```python
from build123d import *

# Parameters (mm, degrees)
F1_DEPTH    = 7.5
F2_W        = 16.1389429122
F2_H        = 16.083650291
F3_DEPTH    = 3
F4_D        = 3.5
F5_T1_DEPTH = 48.2954240112
F6_R        = 5


# Not quite as in the source:
# - a fillet or chamfer that OpenCascade refuses, or shapes differently, is made with other operations: its cross-section is extruded or revolved along the edge and cut away or added


with BuildPart() as f1:
    # F0 (on Top) → F1 (new body)
    with BuildSketch(Plane.XY):
        with BuildLine():
            ThreePointArc((-4.3675557451, -3.9293869513), (0, 5.875), (4.3675557451, -3.9293869513))
            Line((4.3675557451, -3.9293869513), (8.0694714561, -7.2599132545))
            Line((8.0694714561, -7.2599132545), (8.0694714561, 7.2599132545))
            Line((8.0694714561, 7.2599132545), (-8.0694714561, 7.2599132545))
            Line((-8.0694714561, 7.2599132545), (-8.0694714561, -7.2599132545))
            Line((-8.0694714561, -7.2599132545), (-4.3675557451, -3.9293869513))
        make_face()
    extrude(amount=F1_DEPTH)

    # F2 (on face) → F3 (join)
    with BuildSketch(Plane(origin=(0, 7.2599132545, 0), x_dir=(-1, 0, 0), z_dir=(0, 1, 0))):
        with Locations((0, -8.0418251455)):
            Rectangle(F2_W, F2_H)
        with BuildLine():
            Line((1.5, -5.9119383805), (1.5, -11.5))
            ThreePointArc((1.5, -11.5), (0, -13), (-1.5, -11.5))
            Line((-1.5, -11.5), (-1.5, -5.9119383805))
            ThreePointArc((-1.5, -5.9119383805), (0, -4.4119383805), (1.5, -5.9119383805))
        make_face(mode=Mode.SUBTRACT)
        with Locations((0, 8.0418251455)):
            Rectangle(F2_W, F2_H)
    extrude(amount=F3_DEPTH)

    # F4 (through all)
    with Locations(Plane(origin=(0, 7.2599132545, 0), x_dir=(-1, 0, 0), z_dir=(0, -1, 0))):
        with Locations((0, -11.5)):
            Hole(F4_D / 2)

    # F5: fillet of radius 5 on 2 edges, made by hand

    # F5_s2 → F5_t1 (cut)
    with BuildSketch(Plane.XY.offset(-20.3977120056)):
        with BuildLine():
            ThreePointArc((-8.0694714561, 0.8991715477), (-7.0374949846, -2.1429969679), (-4.3675557451, -3.9293869513))
            Line((-4.3675557451, -3.9293869513), (-8.0694714561, -7.2599132545))
            Line((-8.0694714561, -7.2599132545), (-8.0694714561, 0.8991715477))
        make_face()
        with BuildLine():
            ThreePointArc((8.0694714561, 0.8991715477), (7.0374949846, -2.1429969679), (4.3675557451, -3.9293869513))
            Line((4.3675557451, -3.9293869513), (8.0694714561, -7.2599132545))
            Line((8.0694714561, -7.2599132545), (8.0694714561, 0.8991715477))
        make_face()
    extrude(amount=F5_T1_DEPTH, mode=Mode.SUBTRACT)

    # F6
    f6_edges = [f1.edges().sort_by_distance(p)[0] for p in [
        (-8.069471, 8.759913, 16.08365),
        (8.069471, 8.759913, 16.08365),
        (8.069471, 8.759913, -16.08365),
        (-8.069471, 8.759913, -16.08365),
    ]]
    fillet(f6_edges, radius=F6_R)


solid = f1.part
```
Geometry: final body of the model. Coordinates: model frame, mm. A direction names the side the tool comes from. Round coordinates to 2 decimals unless told otherwise and drop trailing zeros. Loops run counter-clockwise (first coordinate to the right, second up) from the corner with the lowest first, then second, coordinate; pieces in that order, holes last. Notation, with made-up numbers: (33, 52) -> (48, 52) arc R26 cw to (48, 86) -> close; hole circle Ø10 at (69, 3.25). An arc over 180 degrees is marked (long way). Write each question's results on one line, items separated by ' | '.
Item 1: Set-up query: faces 1 (the face through (-0.19, 5.87, 3.7)), 2 (the face through (0.033, 8.739, -4.412)), 3 (the face through (-2, 7.26, -8)). Return all of +Z, -Z, +X, -X, +Y, -Y with unobstructed straight access to the full face (end or side cutting, diameter ignored); none if empty.
Answers below:
face 1: +Z, -Z | face 2: +Y, -Y | face 3: -Z, +X, -X, -Y
Item 2: Cut plane A-A on x = 0. Return the cut outline in (y, z) (3 decimals).
Answers below:
outline: (5.875, 0) -> (7.26, 0) -> (7.26, -4.412) -> (10.26, -4.412) -> (10.26, 9.75) -> (7.26, 9.75) -> (7.26, 7.5) -> (5.875, 7.5) -> close; (7.26, -16.084) -> (10.26, -16.084) -> (10.26, -13) -> (7.26, -13) -> close; (7.26, 13.25) -> (10.26, 13.25) -> (10.26, 16.084) -> (7.26, 16.084) -> close
Item 3: Line query: probe 1 along Z at (x, y) = (0, 9.5); probe 2 along Z at (x, y) = (4, 6.5); probe 3 along Y at (x, z) = (2, 13.5). Output: solid intervals per line, ascending. Write a range as [from, to].
Answers below:
probe 1: z = [-16.08, -13], [-4.41, 9.75], [13.25, 16.08] | probe 2: z = [0, 7.5] | probe 3: y = [7.26, 10.26]
Item 4: Pin query (flat end, axial travel): pin 1 Ø5 at (x, y) = (-4.5, -1) entering from -Z; pin 2 Ø4 at (x, z) = (4.5, -8) entering from -Y. Return the tip coordinate at first contact, or that it passes through.
Answers below:
pin 1: stops at z = 0 | pin 2: stops at y = 7.26
Item 5: Cut plane C-C on z = 11.5. Return the cut outline in (x, y), and give its area (3 significant figures).
Answers below:
outline: (-8.05, 7.26) -> (-1.75, 7.26) -> (-1.75, 10.26) -> (-8.05, 10.26) -> close; (1.75, 7.26) -> (8.05, 7.26) -> (8.05, 10.26) -> (1.75, 10.26) -> close | area: 37.8 mm²
Item 6: Cut plane B-B on y = 9.5. Return the cut outline in (x, z), and give its area (3 significant figures).
Answers below:
outline: (-8.07, -11.08) arc R5 ccw to (-3.07, -16.08) -> (3.07, -16.08) arc R5 ccw to (8.07, -11.08) -> (8.07, 11.08) arc R5 ccw to (3.07, 16.08) -> (-3.07, 16.08) arc R5 ccw to (-8.07, 11.08) -> close; hole circle Ø3.5 at (0, 11.5); hole (-1.5, -11.5) arc R1.5 ccw to (1.5, -11.5) -> (1.5, -5.91) arc R1.5 ccw to (-1.5, -5.91) -> close | area: 464 mm²
Item 7: Cut plane D-D on y = 4.25. Return the cut outline in (x, z).
Answers below:
outline: (-8.07, 0) -> (-4.06, 0) -> (-4.06, 7.5) -> (-8.07, 7.5) -> close; (4.06, 0) -> (8.07, 0) -> (8.07, 7.5) -> (4.06, 7.5) -> close
Item 8: Pull-direction query (X, two-part tool) for faces 4 (the face through (-0.228, 8.781, 9.765)), 5 (the face through (-7.065, -2.107, 3.697)), 6 (the face through (2, 7.26, 12)); classes: pulls with the +X half, pulls with the -X half, needs draft (parallel to the pull), parting line crosses it, or undercut.
Answers below:
face 4: undercut | face 5: pulls with the -X half | face 6: needs draft
